Can you work these out from the model? Positions are in its coordinate system, mm. A direction names the side the tool comes from. Round coordinates to 2 decimals unless told otherwise and drop trailing zeros. Order: outer loops, then holes, each group sorted by start corner. A loop starts at its lowest first (then second) coordinate and runs counter-clockwise, first axis right, second up.
from build123d import *

# Parameters (mm, degrees)
SKETCH2_R           = 1
BOSS_EXTRUDE1_DEPTH = 7.5
SKETCH4_W           = 2.6
SKETCH4_H           = 4.1
CUT_EXTRUDE1_DEPTH  = 15
CUT_EXTRUDE3_DEPTH  = 4


with BuildPart() as part:
    # Sketch2 → Boss-Extrude1 (new body, symmetric)
    with BuildSketch(Plane(origin=(0, 0, 0), x_dir=(0, 0, -1), z_dir=(1, 0, 0))):
        with BuildLine():
            Line((-5.018754521, 6.24531137), (-30, 0))
            add(Edge.make_bspline(
                [(-30, 0), (-30, -1.862010614), (-26.296905553, -7.670881077), (-20.233591891, -7.5), (-18, -7.5)],
                knots=[0, 0, 0, 0, 0.469762973, 1, 1, 1, 1], degree=3))
            Line((-18, -7.5), (-11.070367517, -7.5))
            ThreePointArc((-11.070367517, -7.5), (-10.126651666, -7.263349198), (-9.406266928, -6.609400392))
            Line((-9.406266928, -6.609400392), (-2.869582682, 3.195625977))
            ThreePointArc((-2.869582682, 3.195625977), (-2.89885215, 5.457123243), (-5.018754521, 6.24531137))
        make_face()
        with Locations((-4.533683271, 4.30502637)):
            Circle(SKETCH2_R, mode=Mode.SUBTRACT)
        with Locations((-11.070367517, -5.5)):
            Circle(SKETCH2_R, mode=Mode.SUBTRACT)
    extrude(amount=BOSS_EXTRUDE1_DEPTH, both=True)

    # Sketch4 → Cut-Extrude1 (cut)
    with BuildSketch(Plane(origin=(0, 6.30502637, 0), x_dir=(1, 0, 0), z_dir=(0, 1, 0))):
        with Locations((0, -4.583683271)):
            Rectangle(SKETCH4_W, SKETCH4_H)
    extrude(amount=-CUT_EXTRUDE1_DEPTH, mode=Mode.SUBTRACT)

    # Sketch5 → Cut-Extrude3 (cut)
    with BuildSketch(Plane.XZ.offset(7.5)):
        with BuildLine():
            Line((5, 7.070367517), (-5, 7.070367517))
            Line((-5, 7.070367517), (-5, 14.070367517))
            ThreePointArc((-5, 14.070367517), (0, 16.753742727), (5, 14.070367517))
            Line((5, 14.070367517), (5, 7.070367517))
        make_face()
    extrude(amount=-CUT_EXTRUDE3_DEPTH, mode=Mode.SUBTRACT)


solid = part.part
(1) If we mould it in two halves opening along X, with no side actions, what happens to faces 4 (the face through (7.5, -1, 16)), 5 (the face through (0, -3.5, 12)), 6 (the face through (-6.23, -7.27, 10.14)), 7 (the face through (-7.5, -1, 16))? For each: pulls with the +X half, pulls with the -X half, needs draft (parallel to the pull), parting line crosses it, or undercut.
(2) Please list where these lines run through material, in increasing order: probe 1 along X at (y, z) = (-0.5, 6.5); probe 2 along Y at (x, z) = (-7, 4.5); probe 3 along Y at (x, z) = (6.5, 11.75).
(3) I want a section at C-C, the plane y = -5.5. Give the number of separate pieces and of enclosed holes in the cut face, plus the area to 3 significant figures.
(4) I want a section at B-B, the plane z = 15. List the corners of the cut face in (x, y) for me.
(5) I want a section at A-A, the plane z = 6.25. List the corners of the cut face in (x, y) for me (1 decimal), plus the area to 3 significant figures.
(6) I'm going to push flat-ended pins straight in: pin 1 Ø5 at (x, y) = (5, -4.5) entering from +Z; pin 2 Ø1.6 at (y, z) = (-5.5, 11.07) entering from -X; pin 3 Ø2 at (x, y) = (0, 0) entering from -Z; pin 4 Ø6 at (x, z) = (2, 14) entering from +Y. Where does each tip first touch, or does it pass through?
(7) On a 3-axis mill with a long thin cutter (end or side, diameter ignored), from which of +Z, -Z, +X, -X, +Y, -Y can I reach the whole of each face in a straight line? I mean faces 1 (the face through (5, -5.53, 12.25)), 2 (the face through (1.3, 3, 5)), 3 (the face through (6.27, -7.27, 10.14)). Say none if no direction works.
Ans:
1. face 4: pulls with the +X half
1. face 5: undercut
1. face 6: needs draft
1. face 7: pulls with the -X half
2. probe 1: x = -7.5 to -1.3, 1.3 to 7.5
2. probe 2: y = 0.75 to 3.31, 5.3 to 6.3
2. probe 3: y = -7.5 to -6.23, -4.77 to 4.56
3. separate pieces: 3
3. enclosed holes: 0
3. area: 188 mm2
4. outline: (-7.5, -7.5) - (-4.24, -7.5) - (-4.24, -3.5) - (4.24, -3.5) - (4.24, -7.5) - (7.5, -7.5) - (7.5, 3.75) - (-7.5, 3.75) - close
5. outline: (-7.5, -1.9) - (-1.3, -1.9) - (-1.3, 5.9) - (-7.5, 5.9) - close; (1.3, -1.9) - (7.5, -1.9) - (7.5, 5.9) - (1.3, 5.9) - close
5. area: 96.9 mm2
6. pin 1: stops at z = 29.5
6. pin 2: passes through
6. pin 3: stops at z = 6.63
6. pin 4: stops at y = 4.75
7. face 1: -Z, -Y
7. face 2: -Z, +Y, -Y
7. face 3: -Z, +X, -X, -Y
